Here's how the part is built. I have some questions about the finished solid (model axes, mm). A direction names the side the tool comes from. Round coordinates to 2 decimals unless told otherwise and drop trailing zeros. Order: outer loops, then holes, each group sorted by start corner. A loop starts at its lowest first (then second) coordinate and runs counter-clockwise, first axis right, second up. Notation, with made-up numbers: (-15.75, -10.5) -> (26.25, -10.5) arc R16 ccw to (26.25, -4.5) -> close; hole circle Ø5 at (-20, 56.5). An arc over 180 degrees is marked (long way). Answer in a Markdown table with one row per item.
```python
from build123d import *

# Parameters (mm, degrees)
CROQUIS2_R                   = 7.5
CROQUIS2_R_2                 = 4.5
SALIENTE_EXTRUIR1_DEPTH      = 15
REDONDEO2_R                  = 11
CROQUIS4_R                   = 11.5
CORTAR_EXTRUIR1_DEPTH        = 10
TALADRO_DE_MARGEN_PARA_M31_D = 4
MATRIZC1_COUNT               = 4


with BuildPart() as part:
    # Croquis2 → Saliente-Extruir1 (new body)
    with BuildSketch(Plane.XY):
        Polygon((-34.156880773, -21), (34.156880773, -21), (29.048373678, 30), (-29.048373678, 30), align=None)
        with Locations((22, -10)):
            Circle(CROQUIS2_R, mode=Mode.SUBTRACT)
        with Locations((-22, -10)):
            Circle(CROQUIS2_R, mode=Mode.SUBTRACT)
        Circle(CROQUIS2_R_2, mode=Mode.SUBTRACT)
    extrude(amount=SALIENTE_EXTRUIR1_DEPTH)

    # Redondeo2
    redondeo2_edges = [part.edges().sort_by_distance(p)[0] for p in [
        (34.156880773, -21, 7.5),
        (-34.156880773, -21, 7.5),
        (-29.048373678, 30, 7.5),
        (29.048373678, 30, 7.5),
    ]]
    fillet(redondeo2_edges, radius=REDONDEO2_R)

    # Croquis4 → Cortar-Extruir1 (cut)
    with BuildSketch(Plane.XY.offset(15)):
        Circle(CROQUIS4_R)
    extrude(amount=-CORTAR_EXTRUIR1_DEPTH, mode=Mode.SUBTRACT)

    # Taladro de margen para M31 (through all)
    with Locations(Plane(origin=(0, 0, 0), x_dir=(-1, 0, 0), z_dir=(0, 0, -1))):
        with Locations((-5.656854249, 5.656854249)):
            taladro_de_margen_para_m31 = Hole(TALADRO_DE_MARGEN_PARA_M31_D / 2)

    # MatrizC1: Taladro de margen para M31 ×4 about axis
    matrizc1_axis = Axis((0, 0, 0), (0, 0, 1))
    for i in range(1, MATRIZC1_COUNT):
        add(taladro_de_margen_para_m31.rotate(matrizc1_axis, i * 360 / MATRIZC1_COUNT), mode=Mode.SUBTRACT)


solid = part.part
```
1. Suppose I cut it at B-B on y = -10. Write out the boundary of the cut face in (x, z), then the cut area to 3 significant figures.
Numbers:
| item | result |
|---|---|
| outline | (-33, 0) -> (-29.5, 0) -> (-29.5, 15) -> (-33, 15) -> close; (-14.5, 0) -> (14.5, 0) -> (14.5, 15) -> (5.68, 15) -> (5.68, 5) -> (-5.68, 5) -> (-5.68, 15) -> (-14.5, 15) -> close; (29.5, 0) -> (33, 0) -> (33, 15) -> (29.5, 15) -> close |
| area | 426 mm2 |
2. Please list where these lines run through material, in increasing order: line 1 along X through (y, z) = (-15.5, 2.75); line 2 along Y through (x, z) = (0, 1.25); line 3 along X through (y, z) = (-5, 1.5).
Numbers:
| item | result |
|---|---|
| line 1 | x = -31.53 to -27.1, -16.9 to 16.9, 27.1 to 31.53 |
| line 2 | y = -21 to -4.5, 4.5 to 30 |
| line 3 | x = -32.55 to -27.59, -16.41 to -7.55, -3.77 to 3.77, 7.55 to 16.41, 27.59 to 32.55 |
3. Suppose I cut it at C-C on z = 9.75. Write out the boundary of the cut face in (x, y), then the cut area to 3 significant figures.
Numbers:
| item | result |
|---|---|
| outline | (-32.95, -8.9) arc R11 ccw to (-22, -21) -> (22, -21) arc R11 ccw to (32.95, -8.9) -> (30.04, 20.1) arc R11 ccw to (19.1, 30) -> (-19.1, 30) arc R11 ccw to (-30.04, 20.1) -> close; hole circle Ø15 at (-22, -10); hole circle Ø23 at (0, 0); hole circle Ø15 at (22, -10) |
| area | 2,350 mm2 |
4. Suppose I cut it at D-D on y = 0. Write out the boundary of the cut face in (x, z).
Numbers:
| item | result |
|---|---|
| outline | (-32.05, 0) -> (-4.5, 0) -> (-4.5, 5) -> (-11.5, 5) -> (-11.5, 15) -> (-32.05, 15) -> close; (4.5, 0) -> (32.05, 0) -> (32.05, 15) -> (11.5, 15) -> (11.5, 5) -> (4.5, 5) -> close |
5. Suppose I cut it at A-A on x = 0. Write out the boundary of the cut face in (y, z).
Numbers:
| item | result |
|---|---|
| outline | (-21, 0) -> (-4.5, 0) -> (-4.5, 5) -> (-11.5, 5) -> (-11.5, 15) -> (-21, 15) -> close; (4.5, 0) -> (30, 0) -> (30, 15) -> (11.5, 15) -> (11.5, 5) -> (4.5, 5) -> close |
6. We'd pull the mould along X, two halves only. Please class faces 3 (the face through (-29.493, -9.67, 7.395)), 4 (the face through (30.07, -17.475, 7.605)), 5 (the face through (-26.56, 27.08, 7.6)): released by +X, released by -X, zero draft, split by the parting line, or undercut.
Numbers:
| item | result |
|---|---|
| face 3 | undercut |
| face 4 | released by +X |
| face 5 | released by -X |
7. For pin 1 Ø5 at (x, y) = (5.66, 5.66) entering from +Z; pin 2 Ø8 at (y, z) = (-16, 6.5) entering from -X, each with a flat end and sliding along its axis, tell me the tip position at first contact or that it passes through.
Numbers:
| item | result |
|---|---|
| pin 1 | stops at z = 5 |
| pin 2 | stops at x = -32.82 |
8. For faces 1 (the face through (5, 0, 5)), 2 (the face through (26.56, 27.08, 7.6)), which set-ups out of +Z, -Z, +X, -X, +Y, -Y let a thin tool reach every point of the face, with its end or its side?
Numbers:
| item | result |
|---|---|
| face 1 | +Z |
| face 2 | +Z, -Z, +X, +Y |
